from build123d import *

# Parameters (mm, degrees)
CROQUIS1_R                                           = 110.9
SALIENTE_EXTRUIR1_DEPTH                              = 6
CROQUIS2_R                                           = 58.25
CORTAR_EXTRUIR1_DEPTH                                = 6
REFRENTADO_PARA_TORNILLO_CON_CABEZA_TRON_D           = 6.6
REFRENTADO_PARA_TORNILLO_CON_CABEZA_TRON_CBORE_D     = 13
REFRENTADO_PARA_TORNILLO_CON_CABEZA_TRON_CBORE_DEPTH = 4.6
TALADRO_ROSCADO_M6X1_01_D                            = 5


with BuildPart() as part:
    # Croquis1 → Saliente-Extruir1 (new body)
    with BuildSketch(Plane(origin=(0, 0, 0), x_dir=(1, 0, 0), z_dir=(0, 1, 0))):
        with Locations(Location((0, 0, 0), (0, 0, 270))):
            Circle(CROQUIS1_R)
    extrude(amount=SALIENTE_EXTRUIR1_DEPTH)

    # Croquis2 → Cortar-Extruir1 (cut)
    with BuildSketch(Plane(origin=(0, 6, 0), x_dir=(1, 0, 0), z_dir=(0, 1, 0))):
        with Locations(Location((0, 0, 0), (0, 0, 270))):
            Circle(CROQUIS2_R)
    extrude(amount=-CORTAR_EXTRUIR1_DEPTH, mode=Mode.SUBTRACT)

    # Refrentado para tornillo con cabeza troncocónica de M61 (through all)
    with Locations(Plane(origin=(0, 6, 0), x_dir=(1, 0, 0), z_dir=(0, 1, 0))):
        with Locations((-35.304688321, 89.272498467), (23.910965201, 92.974543522), (73.993442721, 61.16347304), (95.812940065, 5.990034727), (81.035150867, -51.471393258), (35.304688321, -89.272498467), (-23.910965201, -92.974543522), (-73.993442721, -61.16347304), (-95.812940065, -5.990034727), (-81.035150867, 51.471393258), (0, 0)):
            CounterBoreHole(REFRENTADO_PARA_TORNILLO_CON_CABEZA_TRON_D / 2, REFRENTADO_PARA_TORNILLO_CON_CABEZA_TRON_CBORE_D / 2, REFRENTADO_PARA_TORNILLO_CON_CABEZA_TRON_CBORE_DEPTH)

    # Taladro roscado M6x1.01 (through all)
    with Locations(Plane(origin=(0, 6, 0), x_dir=(1, 0, 0), z_dir=(0, 1, 0))):
        with Locations((-63.602274198, 17.628122896), (47.067539348, 46.267123746), (16.53473485, -63.895246642), (0, 0)):
            Hole(TALADRO_ROSCADO_M6X1_01_D / 2)


solid = part.part
CAD build for the part. Positions are in the model's coordinates, mm. A direction names the side the tool comes from. Give positions to 0.01 mm unless a question says otherwise; leave off trailing zeros. Order: outer loops, then holes, each group sorted by start corner. A loop starts at its lowest first (then second) coordinate and runs counter-clockwise, first axis right, second up. Notation, with made-up numbers: (54, 13) - (79, 13) arc R16 ccw to (79, 36) - close; hole circle Ø3 at (4, 29.5). An arc over 180 degrees is marked (long way). Answer in a Markdown table with one row per item.
1. Saw through at B-B, the plane y = 4.5. Count the separate pieces of the cut face and the enclosed holes in it, plus the area to 3 significant figures.
Data:
| item | result |
|---|---|
| separate pieces | 1 |
| enclosed holes | 14 |
| area | 26,600 mm² |
2. Pull direction X, two halves, no side cores. Call faces 3 (the cylindrical face through (87.04, 3.73, 53.96)), 4 (the flat face through (-48, 6, 48)): pulls with the +X half, pulls with the -X half, needs draft (parallel to the pull), parting line crosses it, or undercut.
Data:
| item | result |
|---|---|
| face 3 | undercut |
| face 4 | needs draft |
3. Tool access for faces 1 (the flat face through (-76, 1.4, 58)), 2 (the cylindrical face through (72.219, 0.69, -63.946)): list every direction of +Z, -Z, +X, -X, +Y, -Y with a clear straight run to the whole face (end or side of a thin tool).
Data:
| item | result |
|---|---|
| face 1 | +Y |
| face 2 | +Y, -Y |
4. Saw through at A-A, the plane x = 0. Give the cut face in (y, z).
Data:
| item | result |
|---|---|
| outline | (0, -110.9) - (6, -110.9) - (6, -58.25) - (0, -58.25) - close; (0, 58.25) - (6, 58.25) - (6, 110.9) - (0, 110.9) - close |
5. Saw through at C-C, the plane z = 73. Give the cut face in (x, y).
Data:
| item | result |
|---|---|
| outline | (-83.49, 0) - (83.49, 0) - (83.49, 6) - (-83.49, 6) - close |
6. Flat gauge pins, fed straight in: pin 1 (6.5 mm diameter, centred on x = -73, z = 62.5, fed in from +Y); pin 2 (1.5 mm diameter, centred on x = -22, y = 4, fed in from +Z); pin 3 (1.5 mm diameter, centred on y = 3, z = 62.5, fed in from -X). Where does each tip first touch, or does it go through?
Data:
| item | result |
|---|---|
| pin 1 | stops at y = 1.4 |
| pin 2 | stops at z = 108.85 |
| pin 3 | stops at x = -92.12 |
7. Probe probe 1 along X at (y, z) = (5, -95); probe 2 along Z at (x, y) = (40, 1.55); probe 3 along Z at (x, y) = (77, 1.6). List the from-to ranges inside material, lowest first. Write a range as [from, to].
Data:
| item | result |
|---|---|
| probe 1 | x = [-57.22, -38.38], [-32.23, 17.73], [30.09, 57.22] |
| probe 2 | z = [-103.44, -42.34], [42.34, 84.78], [93.77, 103.44] |
| probe 3 | z = [-79.81, -66.93], [-55.4, 46.38], [56.57, 79.81] |
